Could you check a few things on this model? Use its own coordinates, in mm. Face numbers are marked on the shaded views. A direction names the side the tool comes from. Coordinates: 2 decimals unless noted, no trailing zeros. Loops run counter-clockwise (first coordinate to the right, second up) from the corner with the lowest first, then second, coordinate; pieces in that order, holes last. Notation, with made-up numbers: M 52.25,23.5 L 68.25,23.5 A34 ccw 68.25,62.5 Z; hole C -7,-10.5 d9. An arc over 180 degrees is marked long. Write each question's results on one line, items separated by ' | '.
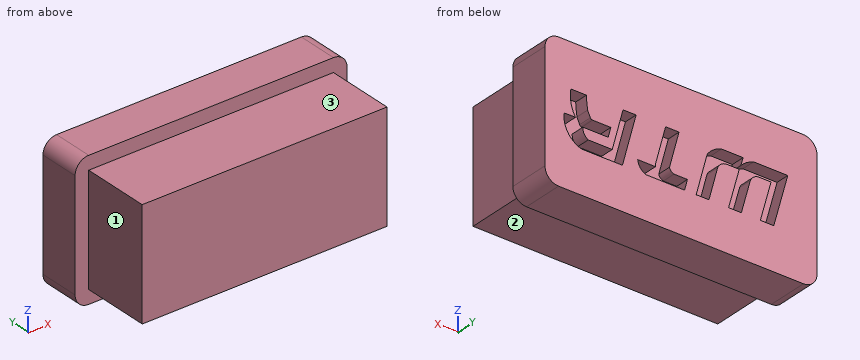
```python
from build123d import *

# Parameters (mm, degrees)
SKETCH_1_W          = 20
SKETCH_1_H          = 10
EXTRUDE_1_DEPTH     = 3
SKETCH_2_W          = 18
SKETCH_2_H          = 8
EXTRUDE_2_DEPTH     = 5
FILLET_1_R          = 1
CUT_EXTRUDE_1_DEPTH = 1


with BuildPart() as part:
    # 草图1 → 凸台-拉伸1 (new body)
    with BuildSketch(Plane(origin=(0, 0, 0), x_dir=(1, 0, 0), z_dir=(0, 1, 0))):
        Rectangle(SKETCH_1_W, SKETCH_1_H)
    extrude(amount=EXTRUDE_1_DEPTH)

    # 草图2 → 凸台-拉伸2 (add)
    with BuildSketch(Plane.XZ):
        Rectangle(SKETCH_2_W, SKETCH_2_H)
    extrude(amount=EXTRUDE_2_DEPTH)

    # 圆角1
    fillet_1_edges = [part.edges().sort_by_distance(p)[0] for p in [
        (10, 1.5, 5),
        (-10, 1.5, 5),
        (-10, 1.5, -5),
        (10, 1.5, -5),
    ]]
    fillet(fillet_1_edges, radius=FILLET_1_R)

    # 草图5 → 切除-拉伸1 (cut)
    with BuildSketch(Plane(origin=(0, 3, 0), x_dir=(1, 0, 0), z_dir=(0, 1, 0))):
        with BuildLine():
            Line((-6.822522061, 1.898386801), (-7.8524835, -1.840514313))
            Line((-7.8524835, -1.840514313), (-5.341070676, -1.840514313))
            ThreePointArc((-5.341070676, -1.840514313), (-4.836499754, -1.613465195), (-4.406580176, -1.265166079))
            Line((-4.406580176, -1.265166079), (-4.565072331, -1.840514313))
            Line((-4.565072331, -1.840514313), (-2.97074846, -1.840514313))
            ThreePointArc((-2.97074846, -1.840514313), (-2.37793404, -1.566363371), (-1.921561777, -1.099124639))
            Line((-1.921561777, -1.099124639), (-1.115765348, 1.898386801))
            Line((-1.115765348, 1.898386801), (-2.05428464, 1.898386801))
            Line((-2.05428464, 1.898386801), (-2.697465694, -0.49420579))
            ThreePointArc((-2.697465694, -0.49420579), (-2.943387046, -0.808990294), (-3.314394459, -0.957044663))
            Line((-3.314394459, -0.957044663), (-4.284751028, -0.957044663))
            Line((-4.284751028, -0.957044663), (-3.498160474, 1.898386801))
            Line((-3.498160474, 1.898386801), (-4.436679766, 1.898386801))
            Line((-4.436679766, 1.898386801), (-5.09577131, -0.49420579))
            ThreePointArc((-5.09577131, -0.49420579), (-5.322706757, -0.801733869), (-5.671922697, -0.957044663))
            Line((-5.671922697, -0.957044663), (-6.621478358, -0.957044663))
            Line((-6.621478358, -0.957044663), (-5.834887804, 1.898386801))
            Line((-5.834887804, 1.898386801), (-6.822522061, 1.898386801))
        make_face()
        with BuildLine():
            Line((-0.475088321, 1.107844934), (-0.262573431, 1.898386801))
            Line((-0.262573431, 1.898386801), (2.578248558, 1.898386801))
            ThreePointArc((2.578248558, 1.898386801), (2.994614434, 1.589766994), (3.185291795, 1.107844934))
            Line((3.185291795, 1.107844934), (1.880601852, 1.107844934))
            Line((1.880601852, 1.107844934), (1.880601852, 0.939138509))
            Line((1.880601852, 0.939138509), (1.13337057, -1.840514313))
            Line((1.13337057, -1.840514313), (0.14506348, -1.840514313))
            Line((0.14506348, -1.840514313), (0.846029375, 0.767034213))
            ThreePointArc((0.846029375, 0.767034213), (0.732607363, 0.989649387), (0.512489482, 1.107844934))
            Line((0.512489482, 1.107844934), (-0.475088321, 1.107844934))
        make_face()
        with BuildLine():
            Line((4.307003713, 1.898386801), (3.301905576, -1.840514313))
            Line((3.301905576, -1.840514313), (4.261825646, -1.840514313))
            Line((4.261825646, -1.840514313), (5.054408893, 1.107844934))
            Line((5.054408893, 1.107844934), (6.821228484, 1.107844934))
            ThreePointArc((6.821228484, 1.107844934), (7.123952053, 0.812017942), (7.213476308, 0.398326541))
            Line((7.213476308, 0.398326541), (5.355376817, 0.398326541))
            Line((5.355376817, 0.398326541), (5.159115285, -0.331753873))
            Line((5.159115285, -0.331753873), (6.505334941, -0.331753873))
            ThreePointArc((6.505334941, -0.331753873), (6.603923501, -0.353634595), (6.670750012, -0.42934911))
            Line((6.670750012, -0.42934911), (6.864004091, -0.875832672))
            ThreePointArc((6.864004091, -0.875832672), (6.92537385, -1.35673953), (6.9569905, -1.840514313))
            Line((6.9569905, -1.840514313), (8.099394952, -1.840514313))
            ThreePointArc((8.099394952, -1.840514313), (8.094576963, -0.91999968), (7.760433181, -0.062259431))
            Line((7.760433181, -0.062259431), (8.581825646, -0.062259431))
            ThreePointArc((8.581825646, -0.062259431), (8.316855125, 1.163927045), (7.299844055, 1.898386801))
            Line((7.299844055, 1.898386801), (4.307003713, 1.898386801))
        make_face()
    extrude(amount=-CUT_EXTRUDE_1_DEPTH, mode=Mode.SUBTRACT)


solid = part.part
```
(1) Imagine slicing it at C-C, the plane z = -3.25. List the corners of the cut face in (x, y) for me, and give its area (3 significant figures).
Reported:
outline: M -10,0 L -9,0 L -9,-5 L 9,-5 L 9,0 L 10,0 L 10,3 L -10,3 Z | area: 150 mm2
(2) Will these pins go through, and if not, where does the flat tip stop? P1, Ø2.5, axis at y = -2, z = 1.5, coming from the +X side; P2, Ø4, axis at x = 0.5, y = -2.5, coming from the -Z side; P3, Ø4, axis at y = -3.5, z = 1.5, coming from the -X side.
Reported:
P1: stops at x = 9 | P2: stops at z = -4 | P3: stops at x = -9
(3) Imagine slicing it at A-A, the plane x = -0.75. List the corners of the cut face in (y, z) for me, and give its area (3 significant figures).
Reported:
outline: M -5,-4 L 0,-4 L 0,-5 L 3,-5 L 3,5 L 0,5 L 0,4 L -5,4 Z | area: 70.0 mm2
(4) Please list where these lines run through material, in increasing order: probe 1 along Z at (x, y) = (7, 2.25); probe 2 along X at (y, z) = (-1.75, -0.25); probe 3 along Z at (x, y) = (-1.5, -3.5). Write a range as from..to.
Reported:
probe 1: z = -5..-1.9, -0.98..-0.4, 1.84..5 | probe 2: x = -9..9 | probe 3: z = -4..4
(5) Which directions (+Z, -Z, +X, -X, +Y, -Y) give clear straight access to the entire face, cutting with the end or side of a thin tool? Please do the marked faces 1, 2 and 3.
Reported:
face 1: +Z, -Z, -X, -Y | face 2: -Z, +X, -X, -Y | face 3: +Z, +X, -X, -Y
(6) Imagine slicing it at B-B, the plane y = 2.25. State how many separate pieces and enclosed holes the cut face has, and give its area (3 significant figures).
Reported:
separate pieces: 1 | enclosed holes: 3 | area: 170 mm2
(7) Imagine slicing it at D-D, the plane y = -0.5. List the corners of the cut face in (x, z) for me.
Reported:
outline: M -9,-4 L 9,-4 L 9,4 L -9,4 Z
